Geometry check sheet. Reference: the model listing, model coordinates, mm. A direction names the side the tool comes from. Round coordinates to 2 decimals unless told otherwise and drop trailing zeros. Order: outer loops, then holes, each group sorted by start corner. A loop starts at its lowest first (then second) coordinate and runs counter-clockwise, first axis right, second up. Notation, with made-up numbers: (-11.75, 63.5) - (1.25, 63.5) arc R18 cw to (1.25, 90.5) - close; hole circle Ø11 at (63, 26). An arc over 180 degrees is marked (long way). Use a Markdown table: item, result. Add a question column.
(1) Thickness scan on line 1 along X through (y, z) = (15.5, 0.5); line 2 along Y through (x, z) = (11.5, -0.25); line 3 along Z through (x, y) = (-10, 37.5). Record the ranges inside material, lowest first. Write a range as [from, to].
(2) Mould release check, pull along Z, two halves, no side actions. Record for faces 1 (the face through (-3.82, 39.43, 5.75)), 2 (the face through (4.452, 20.211, 14.136)), 3 (the face through (-14.084, 20.29, -3.128)), 4 (the face through (-6, 40.996, 0)): released by +Z, released by -Z, zero draft, split by the parting line, or undercut.
(3) Access from +Z, -Z, +X, -X, +Y, -Y to the whole of each face (thin tool, end or side, straight path). Record for faces 5 (the face through (0, 0, 0)), 6 (the face through (0.88, 39.43, -8.83)), 7 (the face through (0, 2.261, 0)).
(4) Section check A-A on z = 7. Record the boundary of the cut face in (x, y).
(5) Gauge pin test, flat ends, axial feed: P1, Ø2, axis at x = -0.18, z = -9.5, coming from the +Y side; P2, Ø10, axis at x = -10, z = -4, coming from the +Y side; P3, Ø1.5, axis at x = 3, y = 48.5, coming from the -Z side; P4, Ø1, axis at y = 30, z = -7.5, coming from the -X side. Record the tip position at first contact, or that the pin passes through.
(6) Section check D-D on z = 10. Record the boundary of the cut face in (x, y), then the cut area to 3 significant figures.
(7) Section check B-B on x = 10.25. Record the boundary of the cut face in (y, z), then the cut area to 3 significant figures.
(8) Section check C-C on y = 34. Record the boundary of the cut face in (x, z), then the cut area to 3 significant figures.
```python
from build123d import *

# Parameters (mm, degrees)
SKETCH1_R           = 14.8209
BOSS_EXTRUDE1_DEPTH = 40.9956
SKETCH2_R           = 5.0165
BOSS_EXTRUDE2_DEPTH = 2.032
SKETCH3_R           = 2.0066
BOSS_EXTRUDE3_DEPTH = 4.1275
SKETCH4_R           = 1.59385
BOSS_EXTRUDE4_DEPTH = 12.0269
FILLET1_R           = 2.54
SKETCH5_R           = 1.25
CUT_EXTRUDE1_DEPTH  = 3.175
SKETCH6_R           = 14.4272
CUT_EXTRUDE2_DEPTH  = 35.56


with BuildPart() as part:
    # Sketch1 → Boss-Extrude1 (new body)
    with BuildSketch(Plane(origin=(0, 0, 0), x_dir=(1, 0, 0), z_dir=(0, 1, 0))):
        with Locations(Location((0, 0, 0), (0, 0, 270))):
            Circle(SKETCH1_R)
    extrude(amount=BOSS_EXTRUDE1_DEPTH)

    # Sketch2 → Boss-Extrude2 (add)
    with BuildSketch(Plane(origin=(0, 40.9956, 0), x_dir=(1, 0, 0), z_dir=(0, 1, 0))):
        with Locations(Location((0, 0, 0), (0, 0, 270))):
            Circle(SKETCH2_R)
    extrude(amount=BOSS_EXTRUDE2_DEPTH)

    # Sketch3 → Boss-Extrude3 (add)
    with BuildSketch(Plane(origin=(0, 43.0276, 0), x_dir=(1, 0, 0), z_dir=(0, 1, 0))):
        with Locations(Location((0, 0, 0), (0, 0, 270))):
            Circle(SKETCH3_R)
    extrude(amount=BOSS_EXTRUDE3_DEPTH)

    # Sketch4 → Boss-Extrude4 (add)
    with BuildSketch(Plane(origin=(0, 47.1551, 0), x_dir=(1, 0, 0), z_dir=(0, 1, 0))):
        with Locations(Location((0, 0, 0), (0, 0, 90))):
            Circle(SKETCH4_R)
    extrude(amount=BOSS_EXTRUDE4_DEPTH)

    # Fillet1
    # the kernel refuses this fillet: 2.54 mm, written as the material it adds along each edge
    with BuildSketch(Plane(origin=(0, 47.1551, 0), x_dir=(0, 0, -1), z_dir=(1, 0, 0))) as fillet1_piece_1:
        with BuildLine():
            CenterArc((4.13385, 1.387950805), FILLET1_R, 180, 33.122940208)
            Line((1.59385, 1.387950805), (1.54305, 1.387950805))
            Line((1.54305, 1.387950805), (1.54305, 0))
            Line((1.54305, 0), (1.59385, -0.0508))
            ThreePointArc((1.59385, -0.0508), (1.800225, -0.0508), (1.964055, -0.027759016))
            Line((1.964055, -0.027759016), (2.0066, 0))
        make_face()
    revolve(axis=Axis((0, 47.1551, 0), (0, 1, 0)))

    # Sketch5 → Cut-Extrude1 (cut)
    with BuildSketch(Plane(origin=(0, 40.9956, 0), x_dir=(1, 0, 0), z_dir=(0, 1, 0))):
        with Locations(Location((-0.175376493, 9.498381077, 0), (0, 0, 270))):
            Circle(SKETCH5_R)
        with Locations(Location((3.871418981, 7.000865309, 0), (0, 0, 270))):
            Circle(SKETCH5_R)
        with Locations(Location((8.138151061, 4.901071037, 0), (0, 0, 270))):
            Circle(SKETCH5_R)
        with Locations(Location((7.998636697, 0.147685468, 0), (0, 0, 270))):
            Circle(SKETCH5_R)
        with Locations(Location((8.313527554, -4.59731004, 0), (0, 0, 270))):
            Circle(SKETCH5_R)
        with Locations(Location((0.175376493, -9.498381077, 0), (0, 0, 270))):
            Circle(SKETCH5_R)
        with Locations(Location((-3.871418981, -7.000865309, 0), (0, 0, 270))):
            Circle(SKETCH5_R)
        with Locations(Location((-8.138151061, -4.901071037, 0), (0, 0, 270))):
            Circle(SKETCH5_R)
        with Locations(Location((-7.998636697, -0.147685468, 0), (0, 0, 270))):
            Circle(SKETCH5_R)
        with Locations(Location((-4.127217715, 6.853179841, 0), (0, 0, 270))):
            Circle(SKETCH5_R)
        with Locations(Location((-8.313527554, 4.59731004, 0), (0, 0, 270))):
            Circle(SKETCH5_R)
        with Locations(Location((4.127217715, -6.853179841, 0), (0, 0, 270))):
            Circle(SKETCH5_R)
    extrude(amount=-CUT_EXTRUDE1_DEPTH, mode=Mode.SUBTRACT)

    # Sketch6 → Cut-Extrude2 (cut)
    with BuildSketch(Plane(origin=(0, 37.8206, 0), x_dir=(1, 0, 0), z_dir=(0, 1, 0))):
        with Locations(Location((0, 0, 0), (0, 0, 270))):
            Circle(SKETCH6_R)
    extrude(amount=-CUT_EXTRUDE2_DEPTH, mode=Mode.SUBTRACT)


solid = part.part
```
Check sheet entries:
| question | item | result |
|---|---|---|
| 1 | line 1 | x = [-14.81, -14.42], [14.42, 14.81] |
| 1 | line 2 | y = [0, 2.26], [37.82, 41] |
| 1 | line 3 | z = [-10.94, -10.4], [10.4, 10.94] |
| 2 | face 1 | undercut |
| 2 | face 2 | split by the parting line |
| 2 | face 3 | undercut |
| 2 | face 4 | zero draft |
| 3 | face 5 | +Z, -Z, +X, -X, -Y |
| 3 | face 6 | +Y |
| 3 | face 7 | none |
| 4 | outline | (-13.06, 0) - (13.06, 0) - (13.06, 41) - (5.37, 41) - (5.37, 37.82) - (12.62, 37.82) - (12.62, 2.26) - (-12.62, 2.26) - (-12.62, 37.82) - (-5.12, 37.82) - (-5.12, 41) - (-13.06, 41) - close; (-2.62, 37.82) - (2.89, 37.82) - (2.89, 41) - (-2.62, 41) - close |
| 5 | P1 | stops at y = 2.26 |
| 5 | P2 | stops at y = 41 |
| 5 | P3 | passes through |
| 5 | P4 | stops at x = -13.06 |
| 6 | outline | (-10.94, 0) - (10.94, 0) - (10.94, 41) - (1.32, 41) - (1.32, 37.82) - (10.4, 37.82) - (10.4, 2.26) - (-10.4, 2.26) - (-10.4, 37.82) - (-0.97, 37.82) - (-0.97, 41) - (-10.94, 41) - close |
| 6 | area | 150 mm2 |
| 7 | outline | (0, -10.7) - (41, -10.7) - (41, 10.7) - (0, 10.7) - close; hole (2.26, -10.15) - (37.82, -10.15) - (37.82, 10.15) - (2.26, 10.15) - close |
| 7 | area | 156 mm2 |
| 8 | outline | circle Ø29.64 at (0, 0); hole circle Ø28.85 at (0, 0) |
| 8 | area | 36.2 mm2 |
